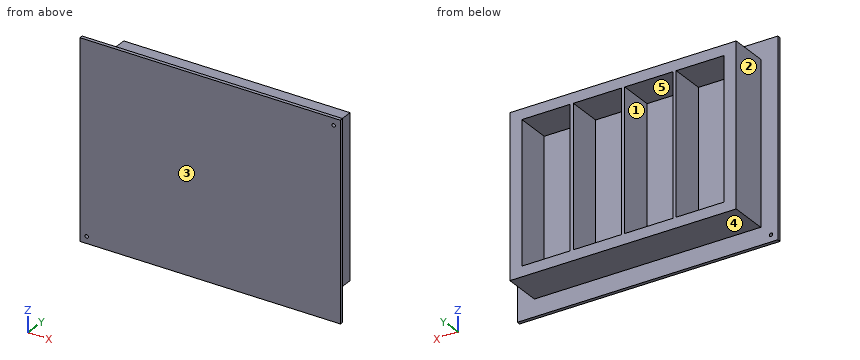
```python
from build123d import *

# Parameters (mm, degrees)
SKETCH1_W           = 66
SKETCH1_H           = 47
SKETCH1_W_2         = 59
SKETCH1_H_2         = 41
BOSS_EXTRUDE1_DEPTH = 10
SKETCH3_W           = 66
SKETCH3_H           = 47
BOSS_EXTRUDE2_DEPTH = 1
SKETCH6_W           = 1
SKETCH6_H           = 41
SKETCH6_W_2         = 0.5
BOSS_EXTRUDE3_DEPTH = 10
SKETCH7_W           = 76
SKETCH7_H           = 57
BOSS_EXTRUDE4_DEPTH = 1
SKETCH8_R           = 0.5
CUT_EXTRUDE1_DEPTH  = 1


with BuildPart() as part:
    # Sketch1 → Boss-Extrude1 (new body)
    with BuildSketch(Plane(origin=(0, 0, 0), x_dir=(1, 0, 0), z_dir=(0, 1, 0))):
        Rectangle(SKETCH1_W, SKETCH1_H)
        Rectangle(SKETCH1_W_2, SKETCH1_H_2, mode=Mode.SUBTRACT)
    extrude(amount=BOSS_EXTRUDE1_DEPTH)

    # Sketch3 → Boss-Extrude2 (add)
    with BuildSketch(Plane(origin=(0, 0, 0), x_dir=(-1, 0, 0), z_dir=(0, -1, 0))):
        Rectangle(SKETCH3_W, SKETCH3_H)
    extrude(amount=BOSS_EXTRUDE2_DEPTH)

    # Sketch6 → Boss-Extrude3 (add)
    with BuildSketch(Plane(origin=(0, 10, 0), x_dir=(1, 0, 0), z_dir=(0, 1, 0))):
        with Locations((-15, 0)):
            Rectangle(SKETCH6_W, SKETCH6_H)
        with Locations((-0.25, 0)):
            Rectangle(SKETCH6_W_2, SKETCH6_H)
        with Locations((0.25, 0)):
            Rectangle(SKETCH6_W_2, SKETCH6_H)
        with Locations((15, 0)):
            Rectangle(SKETCH6_W, SKETCH6_H)
    extrude(amount=-BOSS_EXTRUDE3_DEPTH)

    # Sketch7 → Boss-Extrude4 (add)
    with BuildSketch(Plane(origin=(0, -1, 0), x_dir=(-1, 0, 0), z_dir=(0, -1, 0))):
        Rectangle(SKETCH7_W, SKETCH7_H)
    extrude(amount=BOSS_EXTRUDE4_DEPTH)

    # Sketch8 → Cut-Extrude1 (cut)
    with BuildSketch(Plane(origin=(0, -1, 0), x_dir=(1, 0, 0), z_dir=(0, 1, 0))):
        with Locations(Location((-36, 26.5, 0), (0, 0, 270))):
            Circle(SKETCH8_R)
        with Locations(Location((36, -26.5, 0), (0, 0, 270))):
            Circle(SKETCH8_R)
    extrude(amount=-CUT_EXTRUDE1_DEPTH, mode=Mode.SUBTRACT)


solid = part.part
```
Here's how the part is built. I have some questions about the finished solid (model axes, mm). Face numbers are marked on the shaded views. A direction names the side the tool comes from. Round coordinates to 2 decimals unless told otherwise and drop trailing zeros. Loops run counter-clockwise (first coordinate to the right, second up) from the corner with the lowest first, then second, coordinate; pieces in that order, holes last.
1. Suppose I cut it at C-C, the plane x = -10.5. Please give me the cut outline in (y, z).
Answers:
outline: (-2, -28.5) - (-1, -28.5) - (-1, -23.5) - (10, -23.5) - (10, -20.5) - (0, -20.5) - (0, 20.5) - (10, 20.5) - (10, 23.5) - (-1, 23.5) - (-1, 28.5) - (-2, 28.5) - close
2. Suppose I cut it at B-B, the plane z = -21.5. Please give me the cut outline in (x, y).
Answers:
outline: (-38, -2) - (38, -2) - (38, -1) - (33, -1) - (33, 10) - (-33, 10) - (-33, -1) - (-38, -1) - close
3. Suppose I cut it at A-A, the plane y = 6.5. Please give me the cut outline in (x, z), and give its area (3 significant figures).
Answers:
outline: (-33, -23.5) - (33, -23.5) - (33, 23.5) - (-33, 23.5) - close; hole (-29.5, -20.5) - (-15.5, -20.5) - (-15.5, 20.5) - (-29.5, 20.5) - close; hole (-14.5, -20.5) - (-0.5, -20.5) - (-0.5, 20.5) - (-14.5, 20.5) - close; hole (0.5, -20.5) - (14.5, -20.5) - (14.5, 20.5) - (0.5, 20.5) - close; hole (15.5, -20.5) - (29.5, -20.5) - (29.5, 20.5) - (15.5, 20.5) - close
area: 806 mm2
4. For the marked faces 4 and 5, which set-ups out of +Z, -Z, +X, -X, +Y, -Y let a thin tool reach every point of the face, with its end or its side?
Answers:
face 4: -Z, +X, -X, +Y
face 5: +Y
5. Thinking about a two-plate mould opening in X: for the marked faces 1, 2 and 3, which applies, released by +X, released by -X, zero draft, split by the parting line, or undercut?
Answers:
face 1: undercut
face 2: released by -X
face 3: zero draft
6. Will these pins go through, and if not, where does the flat tip stop? pin 1 (2 mm diameter, centred on x = 24, y = 5.5, fed in from -Z); pin 2 (4 mm diameter, centred on x = 3.5, y = 8.5, fed in from +Z); pin 3 (5 mm diameter, centred on y = 7.5, z = 3.5, fed in from -X).
Answers:
pin 1: stops at z = -23.5
pin 2: stops at z = 23.5
pin 3: stops at x = -33
7. If I drill on probe 1 along Z at (x, y) = (-11.5, 4); probe 2 along X at (y, z) = (3.75, -12); probe 3 along X at (y, z) = (-1.65, 26.5), over which ranges is the centre line in solid material (lowest first)?
Answers:
probe 1: z = -23.5 to -20.5, 20.5 to 23.5
probe 2: x = -33 to -29.5, -15.5 to -14.5, -0.5 to 0.5, 14.5 to 15.5, 29.5 to 33
probe 3: x = -38 to 35.5, 36.5 to 38
8. Suppose I cut it at D-D, the plane z = 14. Please give me the cut outline in (x, y).
Answers:
outline: (-38, -2) - (38, -2) - (38, -1) - (33, -1) - (33, 10) - (29.5, 10) - (29.5, 0) - (15.5, 0) - (15.5, 10) - (14.5, 10) - (14.5, 0) - (0.5, 0) - (0.5, 10) - (-0.5, 10) - (-0.5, 0) - (-14.5, 0) - (-14.5, 10) - (-15.5, 10) - (-15.5, 0) - (-29.5, 0) - (-29.5, 10) - (-33, 10) - (-33, -1) - (-38, -1) - close
